Geometry check sheet. Reference: the model listing, model coordinates, mm. A direction names the side the tool comes from. Coordinates: 2 decimals unless noted, no trailing zeros. Loops run counter-clockwise (first coordinate to the right, second up) from the corner with the lowest first, then second, coordinate; pieces in that order, holes last. Notation, with made-up numbers: (-10.5, 48.25) -> (34.5, 48.25) arc R23 ccw to (34.5, 62.25) -> close; hole circle Ø4 at (55, 25). An arc over 180 degrees is marked (long way). Answer as a JSON object with one key per item and string values.
from build123d import *

# Parameters (mm, degrees)
SKETCH_1_W                    = 480
SKETCH_1_H                    = 94
EXTRUDE_1_DEPTH               = 40
SKETCH_2_W                    = 40
SKETCH_2_H                    = 20
CUT_EXTRUDE_1_DEPTH           = 259.526594377
SKETCH_3_W                    = 360
SKETCH_3_H                    = 20
CUT_EXTRUDE_2_DEPTH           = 259.526594377
SKETCH_4_W                    = 40
SKETCH_4_H                    = 20
CUT_EXTRUDE_3_DEPTH           = 259.526594377
HOLE_WIZARD_M10_1_D           = 11
HOLE_WIZARD_M10_1_CBORE_D     = 18
HOLE_WIZARD_M10_1_CBORE_DEPTH = 11
SKETCH_9_W                    = 385.606218599
SKETCH_9_H                    = 14.697127689
EXTRUDE_2_DEPTH               = 74.29


with BuildPart() as part:
    # 草图1 → 凸台-拉伸1 (new body)
    with BuildSketch(Plane.XZ.offset(20)):
        Rectangle(SKETCH_1_W, SKETCH_1_H)
    extrude(amount=-EXTRUDE_1_DEPTH)

    # 草图2 → 切除-拉伸1 (cut, through all)
    with BuildSketch(Plane(origin=(0, 0, -47), x_dir=(-1, 0, 0), z_dir=(0, 0, -1))):
        with Locations((220, 10)):
            Rectangle(SKETCH_2_W, SKETCH_2_H)
    extrude(amount=-CUT_EXTRUDE_1_DEPTH, mode=Mode.SUBTRACT)

    # 草图3 → 切除-拉伸2 (cut, through all)
    with BuildSketch(Plane(origin=(0, 0, -47), x_dir=(-1, 0, 0), z_dir=(0, 0, -1))):
        with Locations((0, -10)):
            Rectangle(SKETCH_3_W, SKETCH_3_H)
    extrude(amount=-CUT_EXTRUDE_2_DEPTH, mode=Mode.SUBTRACT)

    # 草图4 → 切除-拉伸3 (cut, through all)
    with BuildSketch(Plane(origin=(0, 0, -47), x_dir=(-1, 0, 0), z_dir=(0, 0, -1))):
        with Locations((-220, 10)):
            Rectangle(SKETCH_4_W, SKETCH_4_H)
    extrude(amount=-CUT_EXTRUDE_3_DEPTH, mode=Mode.SUBTRACT)

    # M10 六角头螺栓的柱形沉头孔1 (through all)
    with Locations(Plane(origin=(0, 0, 0), x_dir=(1, 0, 0), z_dir=(0, 1, 0))):
        with Locations((220, -27), (220, 27), (-220, -27), (-220, 27)):
            CounterBoreHole(HOLE_WIZARD_M10_1_D / 2, HOLE_WIZARD_M10_1_CBORE_D / 2, HOLE_WIZARD_M10_1_CBORE_DEPTH)

    # 草图9 → 凸台-拉伸2 (add)
    with BuildSketch(Plane(origin=(0, 20, 0), x_dir=(1, 0, 0), z_dir=(0, 1, 0))):
        with Locations((-0.386766518, -31.52147123)):
            Rectangle(SKETCH_9_W, SKETCH_9_H)
    extrude(amount=EXTRUDE_2_DEPTH)


solid = part.part
1. Mould release check, pull along X, two halves, no side actions. Record for faces 4 (the face through (-240, -10, -1)), 5 (the face through (3, 0, -1)), 6 (the face through (-3, 94.29, 31)), 7 (the face through (-224, -11, -23)): released by +X, released by -X, zero draft, split by the parting line, or undercut.
Evaluation:
{"face 4": "released by -X", "face 5": "undercut", "face 6": "zero draft", "face 7": "undercut"}
2. Section check A-A, the plane z = -27. Record the boundary of the cut face in (x, y), then the cut area to 3 significant figures.
Evaluation:
{"outline": "(-240, -20) -> (-225.5, -20) -> (-225.5, -11) -> (-229, -11) -> (-229, 0) -> (-240, 0) -> close; (-214.5, -20) -> (-180, -20) -> (-180, 0) -> (180, 0) -> (180, -20) -> (214.5, -20) -> (214.5, -11) -> (211, -11) -> (211, 0) -> (200, 0) -> (200, 20) -> (-200, 20) -> (-200, 0) -> (-211, 0) -> (-211, -11) -> (-214.5, -11) -> close; (225.5, -20) -> (240, -20) -> (240, 0) -> (229, 0) -> (229, -11) -> (225.5, -11) -> close", "area": "9,810 mm^2"}
3. Depth check by flat-ended pin: P1, Ø8, axis at x = 153.5, z = 3, coming from the -Y side; P2, Ø1.5, axis at x = 52.5, y = 52.5, coming from the +Z side; P3, Ø9, axis at x = -222.5, z = 25, coming from the +Y side. Enter the tip coordinate at first touch or a pass-through.
Evaluation:
{"P1": "stops at y = 0", "P2": "stops at z = 38.87", "P3": "stops at y = -11"}
4. Section check C-C, the plane x = 60. Record the boundary of the cut face in (y, z).
Evaluation:
{"outline": "(0, -47) -> (20, -47) -> (20, 24.17) -> (94.29, 24.17) -> (94.29, 38.87) -> (20, 38.87) -> (20, 47) -> (0, 47) -> close"}
5. Section check D-D, the plane z = -5. Record the boundary of the cut face in (x, y), then the cut area to 3 significant figures.
Evaluation:
{"outline": "(-240, -20) -> (-180, -20) -> (-180, 0) -> (180, 0) -> (180, -20) -> (240, -20) -> (240, 0) -> (200, 0) -> (200, 20) -> (-200, 20) -> (-200, 0) -> (-240, 0) -> close", "area": "10,400 mm^2"}
6. Tool access check on faces 1 (the face through (180, -10, -1)), 2 (the face through (-220, 0, -1)), 3 (the face through (-3, 57, 24.173)). Record the directions out of +Z, -Z, +X, -X, +Y, -Y that give a thin tool (end or side, any length) a straight path to the whole face; none if there is none.
Evaluation:
{"face 1": "+Z, -Z, -Y", "face 2": "+Z, -Z, -X, +Y", "face 3": "-Z, +X, -X, +Y"}
7. Thickness scan on probe 1 along Z at (x, y) = (220, -13.5); probe 2 along Z at (x, y) = (220, -7.25); probe 3 along X at (y, z) = (-16.5, -27). Record the ranges inside material, lowest first. Write a range as from..to.
Evaluation:
{"probe 1": "z = -47..-32.5, -21.5..21.5, 32.5..47", "probe 2": "z = -47..-36, -18..18, 36..47", "probe 3": "x = -240..-225.5, -214.5..-180, 180..214.5, 225.5..240"}
8. Section check B-B, the plane x = 220. Record the boundary of the cut face in (y, z), then the cut area to 3 significant figures.
Evaluation:
{"outline": "(-20, -47) -> (0, -47) -> (0, -36) -> (-11, -36) -> (-11, -32.5) -> (-20, -32.5) -> close; (-20, -21.5) -> (-11, -21.5) -> (-11, -18) -> (0, -18) -> (0, 18) -> (-11, 18) -> (-11, 21.5) -> (-20, 21.5) -> close; (-20, 32.5) -> (-11, 32.5) -> (-11, 36) -> (0, 36) -> (0, 47) -> (-20, 47) -> close", "area": "1,290 mm^2"}
